Autodesk Inventor part; units mm, degrees
ref_plane "YZ Plane" through (0, 0, 0) normal (1, 0, 0) x (0, 1, 0)
ref_plane "XZ Plane" through (0, 0, 0) normal (0, 1, 0) x (-1, 0, 0)
ref_plane "XY Plane" through (0, 0, 0) normal (0, 0, 1) x (1, 0, 0)
sketch "Sketch1" plane through (0, 0, 0) normal (0, 0, 1) x (1, 0, 0)
  point P0 (0, 0)
sketch "Sketch2" plane through (0, 0, 0) normal (0, 0, 1) x (1, 0, 0)
  line L0 (-12.8291, 6.9625) -> (-12.8291, -14.6342)
  line L1 (-12.8291, -14.6342) -> (291.9709, -14.6342)
  line L2 (291.9709, -14.6342) -> (291.9709, 290.1658)
  line L3 (291.9709, 290.1658) -> (-12.8291, 290.1658)
  line L4 (-12.8291, 290.1658) -> (-12.8291, -14.6342)
  point P0 (0, 0)
  dimension "d0" = 304.8
  dimension "d1" = 304.8
  dimension "d2" = 304.8
  dimension "d3" = 304.8
extrude "Extrusion1" add sketch "Sketch2" along normal blind 304.8
sketch "Sketch3" plane through (0, 0, 304.8) normal (0, 0, 1) x (1, 0, 0)
  line L0 (-1.4082, -1.4082) -> (281.3918, -1.4082)
  line L1 (281.3918, -1.4082) -> (281.3918, 281.3918)
  line L2 (281.3918, 281.3918) -> (-1.4082, 281.3918)
  line L3 (-1.4082, 281.3918) -> (-1.4082, -1.4082)
  line L4 (-1.4082, -1.4082) -> (281.3918, 281.3918) construction
  line L5 (281.3918, -1.4082) -> (-1.4082, 281.3918) construction
  point P0 (0, 0)
  point P1 (139.9918, 139.9918)
  dimension "d8" = 282.8
  dimension "d9" = 282.8
extrude "Extrusion2" cut sketch "Sketch3" against normal blind 302.8
sketch "Sketch4" plane through (0, 0, 2) normal (0, 0, 1) x (1, 0, 0)
  line L0 (-1.4082, 281.3918) -> (281.3918, 281.3918)
  line L1 (120.2104, 281.3918) -> (120.2104, -1.4082)
  line L2 (120.2104, -1.4082) -> (130.8619, -1.4082)
  line L3 (281.3918, -1.4082) -> (-1.4082, -1.4082)
  line L4 (130.8619, -1.4082) -> (130.8619, 281.3918)
  line L5 (130.8619, 281.3918) -> (120.2104, 281.3918)
  line L6 (281.3918, 281.3918) -> (281.3918, -1.4082)
  line L7 (130.8619, 196.2929) -> (281.3918, 196.2929)
  line L8 (281.3918, 196.2929) -> (281.3918, 190.2063)
  line L9 (281.3918, 190.2063) -> (130.8619, 190.2063)
  line L10 (130.8619, 190.2063) -> (130.8619, 196.2929)
  line L11 (130.8619, 88.2557) -> (281.3918, 88.2557)
  line L12 (281.3918, 88.2557) -> (281.3918, 83.6908)
  line L13 (281.3918, 83.6908) -> (130.8619, 83.6908)
  line L14 (130.8619, 83.6908) -> (130.8619, 88.2557)
  line L15 (-1.4082, -1.4082) -> (-1.4082, 281.3918)
  line L16 (-1.4082, 139.9918) -> (120.2104, 139.9918)
  line L17 (120.2104, 139.9918) -> (120.2104, 147.6001)
  line L18 (120.2104, 147.6001) -> (-1.4082, 147.6001)
  line L19 (-1.4082, 147.6001) -> (-1.4082, 139.9918)
  point P0 (0, 0)
  point P1 (-1.4082, 147.6001)
  point P2 (120.2104, 139.9918)
extrude "Extrusion3" add sketch "Sketch4" along normal blind 300 contours L0 L4 L2 L1 | L18 L1 L16 L15 | L7 L6 L9 L4 | L11 L6 L13 L4
sketch "Sketch5" plane through (-1.4082, -1.4082, 304.8) normal (1, 0, 0) x (0, 0, -1)
  line L0 (152.8, 241.4577) -> (224.2375, 241.4577) construction
  line L1 (224.2375, 241.4577) -> (224.2375, 189.864) construction
  line L2 (224.2375, 189.864) -> (152.8, 189.864) construction
  line L3 (152.8, 189.864) -> (152.8, 241.4577) construction
  point P0 (304.8, 1.4082)
sketch "Sketch6" plane through (-1.4082, 281.3918, 304.8) normal (0, -1, 0) x (1, 0, 0)
  line L0 (194.3643, -70.7024) -> (290.2517, -70.7024) construction
  line L1 (290.2517, -70.7024) -> (290.2517, -4.2848) construction
  line L2 (290.2517, -4.2848) -> (194.3643, -4.2848) construction
  line L3 (194.3643, -4.2848) -> (194.3643, -70.7024) construction
  point P0 (1.4082, -304.8)
decal "Decal1"
decal "Decal2"
sketch "Sketch7" plane through (-12.8291, 290.1658, 0) normal (0, 1, 0) x (1, 0, 0)
  circle A0 centre (19.8924, -23.2079) radius 12.1505
  circle A1 centre (269.1255, -23.2079) radius 13.1175
  circle A2 centre (19.8924, -274.4592) radius 7.0633
  circle A3 centre (269.1255, -274.4592) radius 13.1175
  point P0 (12.8291, 0)
sketch "Sketch8" plane through (-12.8291, 290.1658, 0) normal (0, 1, 0) x (1, 0, 0)
  circle A0 centre (18.8833, -266.3869) radius 10.8677
  point P0 (12.8291, 0)
extrude "Extrusion4" add sketch "Sketch8" along normal blind 2
extrude "Extrusion5" add sketch "Sketch7" along normal blind 2 contours A0 | A1 | A3
sketch "Sketch9" plane through (291.9709, -14.6342, 0) normal (1, 0, 0) x (0, 0, -1)
  circle A0 centre (-285.5587, 286.0663) radius 10.8677
  circle A1 centre (-30.2712, 286.0663) radius 11.9817
  circle A2 centre (-30.2712, 39.8602) radius 12.1505
  circle A3 centre (-274.691, 27.7097) radius 12.1505
  point P0 (0, 14.6342)
extrude "Extrusion6" add sketch "Sketch9" along normal blind 2
sketch "Sketch10" plane through (0, 0, 0) normal (0, 0, -1) x (-1, 0, 0)
  circle A0 centre (-270.423, 270.423) radius 11.7673
  circle A1 centre (-16.1447, 270.423) radius 13.2335
  circle A2 centre (-11.0995, 23.208) radius 11.2814
  circle A3 centre (-270.423, 23.208) radius 11.2814
  point P0 (0, 0)
extrude "Extrusion7" add sketch "Sketch10" along normal blind 2
sketch "Sketch11" plane through (-12.8291, -14.6342, 0) normal (0, -1, 0) x (1, 0, 0)
  point P0 (12.8291, 0)
sketch "Sketch12" plane through (-12.8291, -14.6342, 0) normal (0, -1, 0) x (1, 0, 0)
  circle A0 centre (282.2431, 49.443) radius 13.1563
  circle A1 centre (282.2431, 249.2332) radius 13.1563
  circle A2 centre (53.1907, 36.2867) radius 13.5001
  circle A3 centre (39.6907, 249.2332) radius 13.5001
  point P0 (12.8291, 0)
extrude "Extrusion8" add sketch "Sketch12" along normal blind 2
sketch "Sketch13" plane through (-12.8291, -14.6342, 0) normal (-1, 0, 0) x (0, 0, 1)
  circle A0 centre (30.1663, 40.724) radius 12.2858
  circle A1 centre (30.1663, 264.9329) radius 12.0378
  circle A2 centre (256.0059, 264.9329) radius 14.539
  circle A3 centre (264.9742, 23.6025) radius 13.2296
  point P0 (0, 14.6342)
extrude "Extrusion9" add sketch "Sketch13" along normal blind 2
properties part number "locker 2"
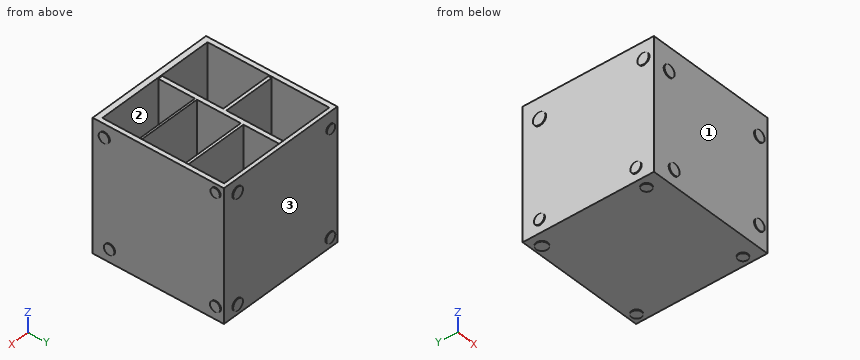
Work out the finished part from the listing and answer in its coordinate system (mm). Face numbers are marked on the shaded views. Coordinates: 2 decimals unless noted, no trailing zeros. Write each loop counter-clockwise with the first axis right and the second up, starting at its lowest first coordinate (ties: lowest second). Pieces come first, ordered by that corner, then holes. Notation, with made-up numbers: (71, 17.25) - (103, 17.25) arc R20 ccw to (103, 45.25) - close; hole circle Ø1 at (74, 76). An arc over 180 degrees is marked (long way). One line per question, with ' | ' between items.
1) Find section B-B, the plane x = 204. Determine the outline of the cut face in (y, z).
Checks:
outline: (-14.63, 0) - (290.17, 0) - (290.17, 304.8) - (281.39, 304.8) - (281.39, 2) - (196.29, 2) - (196.29, 302) - (190.21, 302) - (190.21, 2) - (88.26, 2) - (88.26, 302) - (83.69, 302) - (83.69, 2) - (-1.41, 2) - (-1.41, 304.8) - (-14.63, 304.8) - close
2) Flat-ended cylindrical pins translate along their axes: P1, Ø10, axis at y = 100, z = 134.5, coming from the -X side; P2, Ø10, axis at x = 17, y = 92, coming from the +Z side; P3, Ø1.5, axis at x = 102.5, z = 130.5, coming from the +Y side. Find the tip coordinate at first contact, or state that the pin passes through.
Checks:
P1: x = -12.83 | P2: z = 2 | P3: y = 290.17
3) Find section D-D, the plane x = 83. Determine the outline of the cut face in (y, z).
Checks:
outline: (-14.63, 0) - (290.17, 0) - (290.17, 304.8) - (281.39, 304.8) - (281.39, 2) - (147.6, 2) - (147.6, 302) - (139.99, 302) - (139.99, 2) - (-1.41, 2) - (-1.41, 304.8) - (-14.63, 304.8) - close
4) Find section C-C, the plane y = 229. Determine the outline of the cut face in (x, z), and give its area (3 significant figures).
Checks:
outline: (-12.83, 0) - (291.97, 0) - (291.97, 304.8) - (281.39, 304.8) - (281.39, 2) - (130.86, 2) - (130.86, 302) - (120.21, 302) - (120.21, 2) - (-1.41, 2) - (-1.41, 304.8) - (-12.83, 304.8) - close | area: 10,500 mm2
5) Find section A-A, the plane z = 199. Determine the outline of the cut face in (x, y).
Checks:
outline: (-12.83, -14.63) - (291.97, -14.63) - (291.97, 290.17) - (-12.83, 290.17) - close; hole (-1.41, -1.41) - (120.21, -1.41) - (120.21, 139.99) - (-1.41, 139.99) - close; hole (-1.41, 147.6) - (120.21, 147.6) - (120.21, 281.39) - (-1.41, 281.39) - close; hole (130.86, -1.41) - (281.39, -1.41) - (281.39, 83.69) - (130.86, 83.69) - close; hole (130.86, 88.26) - (281.39, 88.26) - (281.39, 190.21) - (130.86, 190.21) - close; hole (130.86, 196.29) - (281.39, 196.29) - (281.39, 281.39) - (130.86, 281.39) - close
6) The mould has two halves that part along Y. Classify the marked faces 1, 2 and 3: +Y half, -Y half, draft (parallel to the pull), parting line (faces both ways), or undercut.
Checks:
face 1: -Y half | face 2: undercut | face 3: +Y half
7) Consider probe 1 along X at (y, z) = (242.5, 286); probe 2 along Y at (x, z) = (51, 239); probe 3 along Y at (x, z) = (179, 179). Determine where each line is inside the solid, lowest interval first. Write a range as [from, to].
Checks:
probe 1: [-12.83, -1.41], [120.21, 130.86], [281.39, 291.97] | probe 2: [-14.63, -1.41], [139.99, 147.6], [281.39, 290.17] | probe 3: [-14.63, -1.41], [83.69, 88.26], [190.21, 196.29], [281.39, 290.17]
